Model file for the job. Use its own axes, mm. Round coordinates to 2 decimals unless told otherwise and drop trailing zeros. Loops run counter-clockwise (first coordinate to the right, second up) from the corner with the lowest first, then second, coordinate; pieces in that order, holes last. Notation, with made-up numbers: M 68,63.25 L 108,63.25 A22 ccw 108,75.25 Z; hole C 22,-25 d8. An arc over 180 degrees is marked long. Use a Markdown table: item, result. Add a question column.
Item 1: Saw through at D-D on y = -71.5. Write the cut outline in (x, z).
Item 2: Saw through at B-B on y = -101. Write the cut outline in (x, z) (3 decimals).
Item 3: Saw through at A-A on z = 0. Write the cut outline in (x, y).
Item 4: Pin check, flat tips, straight feed: P1, Ø3.5, axis at x = -208, y = -118.5, coming from the +Z side (3 decimals); P2, Ø1, axis at y = -54.5, z = 5, coming from the -X side; P3, Ø4, axis at x = -70.5, z = 4, coming from the -Y side. Stop position of each tip, or through.
Item 5: Saw through at C-C on x = -82.5. Write the cut outline in (y, z).
Item 6: Wall check: L1, parallel to X at y = -81.5, z = -3.25; L2, parallel to X at y = -108, z = -0.5; L3, parallel to Y at x = -22, z = 0.25. Give the ranges that are in metal, low to high. Write a range as from..to.
```python
from build123d import *

# Parameters (mm, degrees)
F0_R      = 6.35
F1_ANGLE  = 90
F2_R      = 6.35
F3_ANGLE  = 90
F4_DEPTH  = 190.5
F5_DEPTH  = 133.35
F6_DEPTH  = 133.35
F8_DEPTH  = 38.1
F11_W     = 26.8649879572
F11_H     = 14.6399100293
F12_DEPTH = 41.275


with BuildPart() as f1:
    # F0 (on Front) → F1 (revolve)
    with BuildSketch(Plane.XZ):
        with Locations((19.05, 0)):
            Circle(F0_R)
    revolve(axis=Axis((0, 0, 21.6534970575), (0, 0, 1)), revolution_arc=F1_ANGLE)

    # F4 (add, through all): a face of the model
    f4_faces = [f1.faces().sort_by_distance(p)[0] for p in [
        (0, 19.05, 0),
    ]]


with BuildPart() as f3:
    # F2 (on Front) → F3 (revolve)
    with BuildSketch(Plane.XZ):
        with Locations((-209.55, 0)):
            Circle(F2_R)
    revolve(axis=Axis((-190.5, 0, 30.7127628475), (0, 0, -1)), revolution_arc=F3_ANGLE)


with BuildPart() as f1_1:
    add(f1.part)

    add(f3.part)  # F4 merges F3
    extrude(f4_faces, amount=F4_DEPTH)

    # F5 (add): a face of the model
    f5_faces = [f1_1.faces().sort_by_distance(p)[0] for p in [
        (19.05, 0, 0),
    ]]
    extrude(f5_faces, amount=F5_DEPTH)

    # F6 (add): a face of the model
    f6_faces = [f1_1.faces().sort_by_distance(p)[0] for p in [
        (-209.55, 0, 0),
    ]]
    extrude(f6_faces, amount=F6_DEPTH)

    # F7 (on face) → F8 (cut)
    with BuildSketch(Plane.XZ.offset(133.35)):
        with BuildLine():
            Line((33.0460654503, 34.1169642213), (-229.9606265432, 34.1169642213))
            Line((-229.9606265432, 34.1169642213), (-229.9606265432, 3.175))
            Line((-229.9606265432, 3.175), (-215.049261314, 3.175))
            ThreePointArc((-215.049261314, 3.175), (-209.55, 6.35), (-204.050738686, 3.175))
            Line((-204.050738686, 3.175), (33.0460654503, 3.175))
            Line((33.0460654503, 3.175), (33.0460654503, 34.1169642213))
        make_face()
    extrude(amount=-F8_DEPTH, mode=Mode.SUBTRACT)

    # F11 (on offset) → F12 (cut)
    with BuildSketch(Plane.XZ.offset(136.525)):
        with Locations((-210.3848606348, 10.4949550146)):
            Rectangle(F11_W, F11_H)
    extrude(amount=-F12_DEPTH, mode=Mode.SUBTRACT)


solid = f1_1.part
```
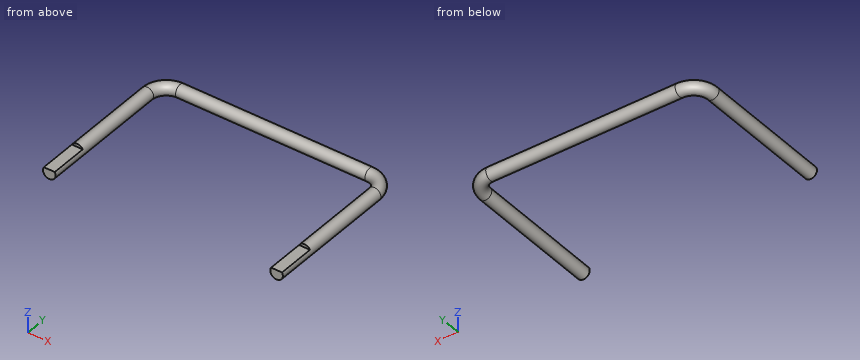
Entries:
| question | item | result |
|---|---|---|
| 1 | outline | C -209.55,0 d12.7; C 19.05,0 d12.7 |
| 2 | outline | M -215.049,3.175 A6.35 ccw long -204.051,3.175 Z; M 13.551,3.175 A6.35 ccw long 24.549,3.175 Z |
| 3 | outline | M -215.9,-133.35 L -203.2,-133.35 L -203.2,0 A12.7 cw -190.5,12.7 L 0,12.7 A12.7 cw 12.7,0 L 12.7,-133.35 L 25.4,-133.35 L 25.4,0 A25.4 ccw 0,25.4 L -190.5,25.4 A25.4 ccw -215.9,0 Z |
| 4 | P1 | z = 3.175 |
| 4 | P2 | x = -214.03 |
| 4 | P3 | y = 13.02 |
| 5 | outline | C 19.05,0 d12.7 |
| 6 | L1 | -215.01..-204.09, 13.59..24.51 |
| 6 | L2 | -215.88..-203.22, 12.72..25.38 |
| 6 | L3 | 12.7..25.4 |
